```python
from build123d import *

# Parameters (mm, degrees)
BOSS_EXTRUDE1_DEPTH = 5.7
SKETCH2_R           = 4
BOSS_EXTRUDE2_DEPTH = 28
SKETCH3_R           = 2
CUT_EXTRUDE1_DEPTH  = 8


with BuildPart() as part:
    # Sketch1 → Boss-Extrude1 (new body)
    with BuildSketch(Plane(origin=(0, 0, 0), x_dir=(1, 0, 0), z_dir=(0, 1, 0))):
        Polygon((0, -7.505553499), (6.5, -3.75277675), (6.5, 3.75277675), (0, 7.505553499), (-6.5, 3.75277675), (-6.5, -3.75277675), align=None)
    extrude(amount=BOSS_EXTRUDE1_DEPTH)

    # Sketch2 → Boss-Extrude2 (add)
    with BuildSketch(Plane(origin=(0, 5.7, 0), x_dir=(1, 0, 0), z_dir=(0, 1, 0))):
        with Locations(Location((0, 0, 0), (0, 0, 270))):
            Circle(SKETCH2_R)
    extrude(amount=BOSS_EXTRUDE2_DEPTH)

    # Sketch3 → Cut-Extrude1 (cut)
    with BuildSketch(Plane(origin=(0, 33.7, 0), x_dir=(1, 0, 0), z_dir=(0, 1, 0))):
        with Locations(Location((0, 0, 0), (0, 0, 270))):
            Circle(SKETCH3_R)
    extrude(amount=-CUT_EXTRUDE1_DEPTH, mode=Mode.SUBTRACT)


solid = part.part
```
For this review, take the finished solid that the model builds, in its own axes (mm). A direction names the side the tool comes from. Coordinates: 2 decimals unless noted, no trailing zeros. Loops run counter-clockwise (first coordinate to the right, second up) from the corner with the lowest first, then second, coordinate; pieces in that order, holes last.
1. Add section D-D, the plane x = 4.5. Give the boundary of the cut face in (y, z).
2. Add section C-C, the plane y = 27. Give the boundary of the cut face in (x, z).
3. For line 1 (X direction, y = 29.5, z = 0); line 2 (Y direction, x = 1.25, z = 0); line 3 (Y direction, x = 5.75, z = 1.25), list the stretches that pass through material, from the lowest coordinate up.
4. Insertion check: P1, Ø2, axis at x = 1, z = -1, coming from the +Y side; P2, Ø3, axis at x = -2, y = 7, coming from the +Z side; P3, Ø1.5, axis at y = 20, z = -2, coming from the -X side; P4, Ø5, axis at x = -2, y = 23.5, coming from the +Z side. Each pin has a flat end and moves straight along its axis. Give the tip position at first contact, or say it passes through.
5. For faces 4 (the flat face through (-1, 33.7, -2)), 5 (the cylindrical face through (-3.905, 19.504, -0.867)), list the 3-axis set-ups (+Z, -Z, +X, -X, +Y, -Y) from which the entire face can be reached by the end or side of a thin tool; tool diameter is ignored.
6. Mouldability with a two-part tool opening along Z and no side actions: class faces 1 (the flat face through (0, 25.7, 0)), 2 (the flat face through (-3.2, 2.81, -5.66)), 3 (the flat face through (3, 5.7, 3)) as +Z half, -Z half, draft (parallel to the pull), parting line (faces both ways), or undercut.
7. Add section B-B, the plane y = 4.5. Give the boundary of the cut face in (x, z).
8. Add section A-A, the plane z = 0. Give the boundary of the cut face in (x, y).
Result:
1. outline: (0, -4.91) - (5.7, -4.91) - (5.7, 4.91) - (0, 4.91) - close
2. outline: circle Ø8 at (0, 0); hole circle Ø4 at (0, 0)
3. line 1: x = -4 to -2, 2 to 4
3. line 2: y = 0 to 25.7
3. line 3: y = 0 to 5.7
4. P1: stops at y = 33.7
4. P2: stops at z = 6.78
4. P3: stops at x = -3.8
4. P4: stops at z = 4
5. face 4: +Z, -Z, +X, -X, +Y
5. face 5: +Y
6. face 1: undercut
6. face 2: -Z half
6. face 3: draft
7. outline: (-6.5, -3.75) - (0, -7.51) - (6.5, -3.75) - (6.5, 3.75) - (0, 7.51) - (-6.5, 3.75) - close
8. outline: (-6.5, 0) - (6.5, 0) - (6.5, 5.7) - (4, 5.7) - (4, 33.7) - (2, 33.7) - (2, 25.7) - (-2, 25.7) - (-2, 33.7) - (-4, 33.7) - (-4, 5.7) - (-6.5, 5.7) - close
